```python
from build123d import *

# Parameters (mm, degrees)
SKETCH_1_R      = 1.5
EXTRUDE_1_DEPTH = 4
FILLET_1_R      = 15


with BuildPart() as part:
    # 草图1 → 凸台-拉伸1 (new body)
    with BuildSketch(Plane.XY):
        with BuildLine():
            Line((-3, 15), (-3, 1.732050808))
            Line((-3, 1.732050808), (-14.490381057, -4.901923789))
            ThreePointArc((-14.490381057, -4.901923789), (-15.588457268, -9), (-11.490381057, -10.098076211))
            Line((-11.490381057, -10.098076211), (0, -3.464101615))
            Line((0, -3.464101615), (11.490381057, -10.098076211))
            ThreePointArc((11.490381057, -10.098076211), (15.588457268, -9), (14.490381057, -4.901923789))
            Line((14.490381057, -4.901923789), (3, 1.732050808))
            Line((3, 1.732050808), (3, 15))
            ThreePointArc((3, 15), (0, 18), (-3, 15))
        make_face()
        with Locations((0, 15)):
            Circle(SKETCH_1_R, mode=Mode.SUBTRACT)
        with Locations((12.990381057, -7.5)):
            Circle(SKETCH_1_R, mode=Mode.SUBTRACT)
        with Locations((-12.990381057, -7.5)):
            Circle(SKETCH_1_R, mode=Mode.SUBTRACT)
    extrude(amount=EXTRUDE_1_DEPTH)

    # 圆角1
    fillet_1_edges = [part.edges().sort_by_distance(p)[0] for p in [
        (-3, 1.732050808, 2),
        (3, 1.732050808, 2),
        (0, -3.464101615, 2),
    ]]
    fillet(fillet_1_edges, radius=FILLET_1_R)


solid = part.part
```
Check sheet for the modelled part. Datum: model origin and axes. Units: mm. A direction names the side the tool comes from. Give positions to 0.01 mm unless a question says otherwise; leave off trailing zeros. Loops run counter-clockwise (first coordinate to the right, second up) from the corner with the lowest first, then second, coordinate; pieces in that order, holes last. Notation, with made-up numbers: M 49.5,-10 L 61.5,-10 A20 cw 61.5,10 Z; hole C -36,81.5 d10. An arc over 180 degrees is marked long. Answer in a Markdown table with one row per item.
1) Depth check by flat-ended pin: pin 1 (1.5 mm diameter, centred on x = 5.5, y = 14, fed in from +Z); pin 2 (2 mm diameter, centred on y = 13, z = 3.5, fed in from -X). Enter the tip coordinate at first touch or a pass-through.
Solutions:
| item | result |
|---|---|
| pin 1 | passes through |
| pin 2 | stops at x = -3 |
2) Thickness scan on line 1 (Y direction, x = 0, z = 3.15); line 2 (X direction, y = -8.75, z = 1.85); line 3 (X direction, y = -8.5, z = 1.4). Record the ranges inside material, lowest first.
Solutions:
| item | result |
|---|---|
| line 1 | y = -5.78 to 13.5, 16.5 to 18 |
| line 2 | x = -15.72 to -13.82, -12.16 to -9.16, 9.16 to 12.16, 13.82 to 15.72 |
| line 3 | x = -15.82 to -14.11, -11.87 to -8.72, 8.72 to 11.87, 14.11 to 15.82 |
3) Cross-section at D-D (x = -8.5). Enter the section's corners in (y, z), plus the area to 3 significant figures.
Solutions:
| item | result |
|---|---|
| outline | M -8.37,0 L -1.22,0 L -1.22,4 L -8.37,4 Z |
| area | 28.6 mm^2 |
4) Mould release check, pull along Y, two halves, no side actions. Record for faces 1 (the face through (-14.181, -8.413, 1.972)), 2 (the face through (-1.11, 16.01, 1.97)), 3 (the face through (-12.467, -3.734, 1.972)), 4 (the face through (-0.11, -5.785, 2.028)): released by +Y, released by -Y, zero draft, split by the parting line, or undercut.
Solutions:
| item | result |
|---|---|
| face 1 | undercut |
| face 2 | undercut |
| face 3 | released by +Y |
| face 4 | released by -Y |
5) Cross-section at B-B (z = 1.55). Enter the section's corners in (x, y), plus the area to 3 significant figures.
Solutions:
| item | result |
|---|---|
| outline | M -14.49,-4.9 A3 ccw -11.49,-10.1 L -7.5,-7.79 A15 cw 7.5,-7.79 L 11.49,-10.1 A3 ccw 14.49,-4.9 L 10.5,-2.6 A15 cw 3,10.39 L 3,15 A3 ccw -3,15 L -3,10.39 A15 cw -10.5,-2.6 Z; hole C -12.99,-7.5 d3; hole C 0,15 d3; hole C 12.99,-7.5 d3 |
| area | 312 mm^2 |
6) Cross-section at C-C (y = -2.25). Enter the section's corners in (x, z), plus the area to 3 significant figures.
Solutions:
| item | result |
|---|---|
| outline | M -9.93,0 L 9.93,0 L 9.93,4 L -9.93,4 Z |
| area | 79.4 mm^2 |
7) Tool access check on faces 5 (the face through (3, 13, 2)), 6 (the face through (9.47, -8.93, 1.97)), 7 (the face through (13.68, -8.83, 1.97)), 8 (the face through (-3, 13, 2)). Record the directions out of +Z, -Z, +X, -X, +Y, -Y that give a thin tool (end or side, any length) a straight path to the whole face; none if there is none.
Solutions:
| item | result |
|---|---|
| face 5 | +Z, -Z, +X, +Y |
| face 6 | +Z, -Z, -Y |
| face 7 | +Z, -Z |
| face 8 | +Z, -Z, -X, +Y |
8) Cross-section at A-A (x = 0). Enter the section's corners in (y, z), plus the area to 3 significant figures.
Solutions:
| item | result |
|---|---|
| outline | M -5.78,0 L 13.5,0 L 13.5,4 L -5.78,4 Z; M 16.5,0 L 18,0 L 18,4 L 16.5,4 Z |
| area | 83.1 mm^2 |
